from build123d import *

# Parameters (mm, degrees)
F0_W           = 160
F0_H           = 100
F0_R           = 6
F0_W_2         = 78
F0_H_2         = 64
F1_DEPTH       = 25
F2_W           = 78
F2_H           = 64
F3_DEPTH       = 625
F5_DEPTH       = 26
F6_W           = 80
F6_H           = 100
F7_DEPTH       = 15
F9_DEPTH       = 22
F11_D          = 4.2
F11_DEPTH      = 10.4
F11_TIP        = 1.2618073
F13_DEPTH      = 20
F15_DEPTH      = 21
F17_DEPTH      = 525
F17_DEPTH_BACK = 3
F18_R          = 1.24999


# Not quite as in the source:
# - a fillet or chamfer is up to 0.001 mm smaller than in the source, because OpenCascade refuses the exact size


with BuildPart() as f1:
    # F0 (on Top) → F1 (new body)
    with BuildSketch(Plane.XY):
        Rectangle(F0_W, F0_H)
        with Locations((-65, -30)):
            Circle(F0_R, mode=Mode.SUBTRACT)
        with Locations((65, -30)):
            Circle(F0_R, mode=Mode.SUBTRACT)
        with Locations((-65, 30)):
            Circle(F0_R, mode=Mode.SUBTRACT)
        with Locations((0, 8)):
            Rectangle(F0_W_2, F0_H_2, mode=Mode.SUBTRACT)
        with Locations((65, 30)):
            Circle(F0_R, mode=Mode.SUBTRACT)
    extrude(amount=F1_DEPTH)

    # F2 (on face) → F3 (join)
    with BuildSketch(Plane.XY.offset(25)):
        Polygon((50, 50), (-50, 50), (-50, -13), (-60, -23), (-60, -35), (-27.3397459622, -35), (-36, -50), (44, -50), (35.3397459622, -35), (60, -35), (60, -23), (50, -13), align=None)
        with Locations((0, 8)):
            Rectangle(F2_W, F2_H, mode=Mode.SUBTRACT)
    extrude(amount=F3_DEPTH)

    # F4 (on face) → F5 (cut, through all)
    with BuildSketch(Plane.XZ.offset(50)):
        with BuildLine():
            ThreePointArc((-18, 193), (0, 175), (18, 193))
            Line((18, 193), (18, 587))
            ThreePointArc((18, 587), (0, 605), (-18, 587))
            Line((-18, 587), (-18, 193))
        make_face()
    extrude(amount=-F5_DEPTH, mode=Mode.SUBTRACT)

    # F6 (on face) → F7 (cut, through all)
    with BuildSketch(Plane.XZ.offset(50)):
        with Locations((4, 75)):
            Rectangle(F6_W, F6_H)
    extrude(amount=-F7_DEPTH, mode=Mode.SUBTRACT)

    # F8 (on face) → F9 (cut, through all)
    with BuildSketch(Plane.XZ.offset(35)):
        Polygon((-60, 75), (-60, 25), (-50, 25), (-50, 65), align=None)
        Polygon((50, 65), (50, 25), (60, 25), (60, 75), align=None)
    extrude(amount=-F9_DEPTH, mode=Mode.SUBTRACT)

    # F11
    with Locations(Plane.XY.offset(650)):
        with Locations((-41, 43.5), (41, 43.5), (41, -28.5), (-41, -28.5)):
            Hole(F11_D / 2, depth=F11_DEPTH)
            with Locations((0, 0, -(F11_DEPTH + F11_TIP / 2))):  # 118° drill point
                Cone(0, F11_D / 2, F11_TIP, mode=Mode.SUBTRACT)

    # F12 (on face) → F13 (join)
    with BuildSketch(Plane.XY.offset(650)):
        with BuildLine():
            Line((-39, 40), (-39, 28.6339312527))
            ThreePointArc((-39, 28.6339312527), (-30.9466258481, 32.367629715), (-26.4140478542, 40))
            Line((-26.4140478542, 40), (-39, 40))
        make_face()
        with BuildLine():
            Line((39, 40), (26.4140478542, 40))
            ThreePointArc((26.4140478542, 40), (30.9466258481, 32.367629715), (39, 28.6339312527))
            Line((39, 28.6339312527), (39, 40))
        make_face()
        with BuildLine():
            ThreePointArc((-26.6909119787, -24), (-31.3376797124, -17.0265712771), (-39, -13.6339312527))
            Line((-39, -13.6339312527), (-39, -24))
            Line((-39, -24), (-26.6909119787, -24))
        make_face()
        with BuildLine():
            ThreePointArc((39, -13.6339312527), (31.3376797124, -17.0265712771), (26.6909119787, -24))
            Line((26.6909119787, -24), (39, -24))
            Line((39, -24), (39, -13.6339312527))
        make_face()
    extrude(amount=-F13_DEPTH)

    # F14 (on face) → F15 (cut, through all)
    with BuildSketch(Plane.YZ.offset(60)):
        with BuildLine():
            Line((35, 630), (-23, 630))
            Line((-23, 630), (-23, 530))
            Line((-23, 530), (35, 530))
            ThreePointArc((35, 530), (38.5355339059, 531.4644660941), (40, 535))
            Line((40, 535), (40, 625))
            ThreePointArc((40, 625), (38.5355339059, 628.5355339059), (35, 630))
        make_face()
        with BuildLine():
            Line((-23, 630), (-25, 630))
            ThreePointArc((-25, 630), (-28.5355339059, 628.5355339059), (-30, 625))
            Line((-30, 625), (-30, 535))
            ThreePointArc((-30, 535), (-28.5355339059, 531.4644660941), (-25, 530))
            Line((-25, 530), (-23, 530))
            Line((-23, 530), (-23, 630))
        make_face()
    extrude(amount=-F15_DEPTH, mode=Mode.SUBTRACT)

    # F16 (on face) → F17 (cut, two sides)
    with BuildSketch(Plane(origin=(0, 0, 125), x_dir=(1, 0, 0), z_dir=(0, 0, -1))) as f17_sk:
        Polygon((36.5897459622, 37.1650635095), (34.7147459622, 36.0825317547), (35.9647459622, 33.9174682453), (37.8397459622, 35), align=None)
        Polygon((-27.9647459622, 33.9174682453), (-26.7147459622, 36.0825317547), (-28.5897459622, 37.1650635095), (-29.8397459622, 35), align=None)
    extrude(amount=-F17_DEPTH, mode=Mode.SUBTRACT)
    extrude(f17_sk.sketch, amount=F17_DEPTH_BACK, mode=Mode.SUBTRACT)

    # F18 (radius 1.25 in the source; OpenCascade refuses exactly that, so slightly less here)
    f18_edges = [f1.edges().sort_by_distance(p)[0] for p in [
        (36.902246, -34.458734, 122),
        (-28.902246, -34.458734, 122),
    ]]
    fillet(f18_edges, radius=F18_R)


solid = f1.part
CAD build for the part. Positions are in the model's coordinates, mm. A direction names the side the tool comes from. Coordinates: 2 decimals unless noted, no trailing zeros. Write each loop counter-clockwise with the first axis right and the second up, starting at its lowest first coordinate (ties: lowest second). Pieces come first, ordered by that corner, then holes. Notation, with made-up numbers: (80, 34) - (114, 34) arc R25 cw to (114, 53) - close; hole circle Ø6 at (81.25, 10.5). An arc over 180 degrees is marked (long way). Use a Markdown table: item, result. Add a question column.
Item 1: Drill centre lines: L1, parallel to Y at x = 65, z = 12; L2, parallel to X at y = -28, z = 643; L3, parallel to Z at x = -1.5, y = -40.5. Where is each one in solid material? Low to high. Write a range as from..to.
Item 2: Band-saw the part on A-A, the plane y = -3. Give the cut face in (x, z), and give its area (3 significant figures).
Item 3: Band-saw the part on C-C, the plane z = 53. Give the cut face in (x, y).
Item 4: Band-saw the part on D-D, the plane z = 317.5. Give the cut face in (x, y), and give its area (3 significant figures).
Item 5: 3-axis set-ups, long thin cutter, end or side, ignore diameter. For faces 4 (the face through (30.853, 32.453, 640.14)), 5 (the face through (-27, -24, 320)), 6 (the face through (3, -43, 125)): which of +Z, -Z, +X, -X, +Y, -Y reach the whole face in a straight line?
Item 6: Flat gauge pins, fed straight in: pin 1 (8 mm diameter, centred on y = -39.5, z = 470, fed in from -X); pin 2 (3 mm diameter, centred on y = -15.5, z = 123, fed in from +X); pin 3 (8 mm diameter, centred on y = -40.5, z = 366.5, fed in from +X). Where does each tip first touch, or does it go through?
Item 7: Mould opens along Z. For faces 1 (the face through (-1, -33, 650)), 2 (the face through (43, 1, 630)), 3 (the face through (-31.25, -17.1, 640.14)) say: pulls with the +Z half, pulls with the -Z half, needs draft (parallel to the pull), parting line crosses it, or undercut.
Item 8: Band-saw the part on B-B, the plane x = 0. Give the cut face in (y, z).
Numbers:
| question | item | result |
|---|---|---|
| 1 | L1 | -50..-36, -24..24, 36..50 |
| 1 | L2 | -60..-43.04, -38.96..38.96, 43.04..60 |
| 1 | L3 | 0..25, 125..175.06, 604.94..650 |
| 2 | outline | (-80, 0) - (-39, 0) - (-39, 650) - (-50, 650) - (-50, 25) - (-80, 25) - close; (39, 0) - (80, 0) - (80, 25) - (50, 25) - (50, 530) - (39, 530) - close; (39, 630) - (50, 630) - (50, 650) - (39, 650) - close |
| 2 | area | 14,700 mm2 |
| 3 | outline | (-50, -35) - (50, -35) - (50, 50) - (-50, 50) - close; hole (-39, -24) - (39, -24) - (39, 40) - (-39, 40) - close |
| 4 | outline | (-60, -35) - (-29.84, -35) - (-27.96, -33.92) - (-26.71, -36.08) - (-28.59, -37.17) - (-36, -50) - (-18, -50) - (-18, -24) - (-39, -24) - (-39, 40) - (39, 40) - (39, -24) - (18, -24) - (18, -50) - (44, -50) - (36.59, -37.17) - (34.71, -36.08) - (35.96, -33.92) - (37.84, -35) - (60, -35) - (60, -23) - (50, -13) - (50, 50) - (-50, 50) - (-50, -13) - (-60, -23) - close |
| 4 | area | 3,980 mm2 |
| 5 | face 4 | +Z, -Z |
| 5 | face 5 | -Z |
| 5 | face 6 | +X, -X, -Y |
| 6 | pin 1 | x = -32.25 |
| 6 | pin 2 | x = 54 |
| 6 | pin 3 | x = 40.82 |
| 7 | face 1 | pulls with the +Z half |
| 7 | face 2 | undercut |
| 7 | face 3 | needs draft |
| 8 | outline | (-50, 0) - (-24, 0) - (-24, 175) - (-50, 175) - (-50, 125) - (-35, 125) - (-35, 25) - (-50, 25) - close; (-50, 605) - (-24, 605) - (-24, 650) - (-50, 650) - close; (40, 0) - (50, 0) - (50, 650) - (40, 650) - close |
